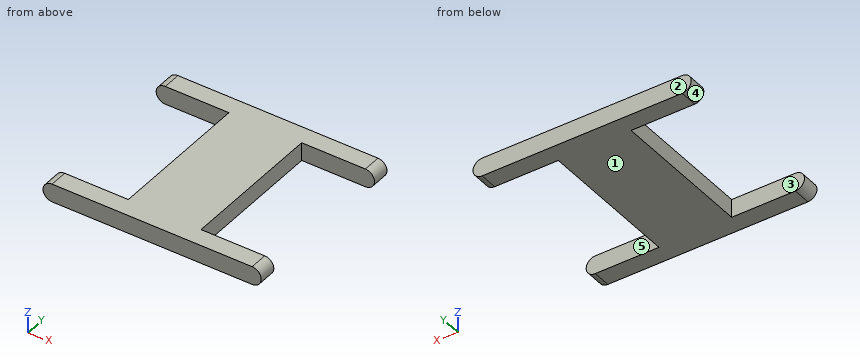
```python
from build123d import *

# Parameters (mm, degrees)
EXTRUDE_1_DEPTH     = 20
SKETCH_2_W          = 8
SKETCH_2_H          = 16
CUT_EXTRUDE_1_DEPTH = 12


with BuildPart() as part:
    # 草图1 → 凸台-拉伸1 (new body)
    with BuildSketch(Plane(origin=(0, 0, 0), x_dir=(1, 0, 0), z_dir=(0, 1, 0))):
        with BuildLine():
            Line((-11, 1), (11, 1))
            ThreePointArc((11, 1), (12, 0), (11, -1))
            Line((11, -1), (-11, -1))
            ThreePointArc((-11, -1), (-12, 0), (-11, 1))
        make_face()
    extrude(amount=EXTRUDE_1_DEPTH)

    # 草图2 → 切除-拉伸1 (cut)
    with BuildSketch(Plane(origin=(0, 0, -1), x_dir=(-1, 0, 0), z_dir=(0, 0, -1))):
        with Locations((-8, 10)):
            Rectangle(SKETCH_2_W, SKETCH_2_H)
        with Locations((8, 10)):
            Rectangle(SKETCH_2_W, SKETCH_2_H)
    extrude(amount=-CUT_EXTRUDE_1_DEPTH, mode=Mode.SUBTRACT)


solid = part.part
```
The listing builds one solid part. Answer for the finished solid, in the listing's coordinates (mm). Face numbers are marked on the shaded views. A direction names the side the tool comes from. Round coordinates to 2 decimals unless told otherwise and drop trailing zeros. Loops run counter-clockwise (first coordinate to the right, second up) from the corner with the lowest first, then second, coordinate; pieces in that order, holes last. Notation, with made-up numbers: (-14, 85.25) -> (-3, 85.25) arc R11 cw to (-3, 95.25) -> close; hole circle Ø7 at (-0.75, 52.25). An arc over 180 degrees is marked (long way). Use one line per item in the form item = value.
1. The part is cut by section B-B on z = 0. Determine the outline of the cut face in (x, y), and give its area (3 significant figures).
Answer key:
outline = (-12, 0) -> (12, 0) -> (12, 2) -> (4, 2) -> (4, 18) -> (12, 18) -> (12, 20) -> (-12, 20) -> (-12, 18) -> (-4, 18) -> (-4, 2) -> (-12, 2) -> close
area = 224 mm²
2. A flat-ended cylindrical pin translates along its axis: pin 1 Ø0.6 at (y, z) = (11, 0.5) entering from +X. Find the tip coordinate at first contact, or state that the pin passes through.
Answer key:
pin_1 = 4
3. The part is cut by section A-A on x = 7.5. Determine the outline of the cut face in (y, z), and give its area (3 significant figures).
Answer key:
outline = (0, -1) -> (2, -1) -> (2, 1) -> (0, 1) -> close; (18, -1) -> (20, -1) -> (20, 1) -> (18, 1) -> close
area = 8.00 mm²
4. The part is cut by section C-C on y = 18.5. Determine the outline of the cut face in (x, z).
Answer key:
outline = (-11, -1) -> (11, -1) arc R1 ccw to (11, 1) -> (-11, 1) arc R1 ccw to start
5. A tool of negligible diameter and unlimited length cuts with its end or side. For the marked faces 4 and 5, from which of +Z, -Z, +X, -X, +Y, -Y can it reach the whole face along a straight path? Write none if from no direction.
Answer key:
face_4 = -X, +Y, -Y
face_5 = +Z, -Z, +X
6. The part is cut by section D-D on y = 14.25. Determine the outline of the cut face in (x, z).
Answer key:
outline = (-4, -1) -> (4, -1) -> (4, 1) -> (-4, 1) -> close
7. Find the intervals of material crossed by probe 1 along Y at (x, z) = (-6, -0.25); probe 2 along X at (y, z) = (6.5, -0.75), in increasing order. Write a range as [from, to].
Answer key:
probe_1 = [0, 2], [18, 20]
probe_2 = [-4, 4]
8. For a pull along Y with two mould halves and no side action, classify the marked faces 1, 2 and 3 as released by +Y, released by -Y, zero draft, split by the parting line, or undercut.
Answer key:
face_1 = zero draft
face_2 = released by +Y
face_3 = undercut
